For this review, take the finished solid that the model builds, in its own axes (mm). Face numbers are marked on the shaded views. A direction names the side the tool comes from. Give positions to 0.01 mm unless a question says otherwise; leave off trailing zeros. Loops run counter-clockwise (first coordinate to the right, second up) from the corner with the lowest first, then second, coordinate; pieces in that order, holes last. Notation, with made-up numbers: (4.5, 69.5) - (30.5, 69.5) arc R25 cw to (30.5, 81.5) - close; hole circle Ø2 at (23, 86). An arc over 180 degrees is marked (long way). Put each result on its own line as item: value. Start each with the question number.
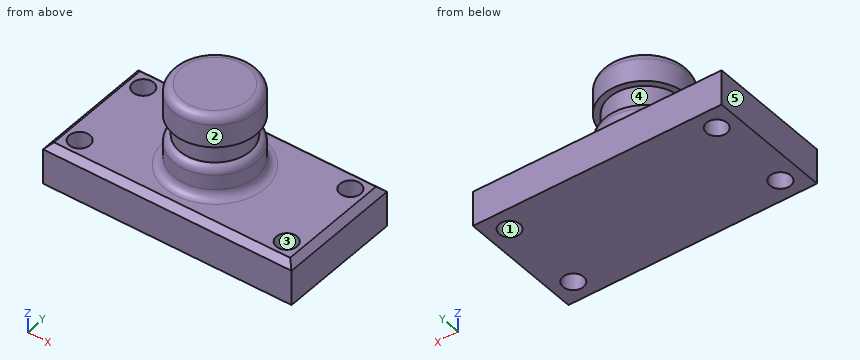
from build123d import *

# Parameters (mm, degrees)
F0_W     = 152.4
F0_H     = 76.2
F1_DEPTH = 25.4
F2_R     = 6.35
F3_DEPTH = 25.401
F4_SIZE  = 3.81


# Not quite as in the source:
# - a fillet or chamfer that OpenCascade refuses, or shapes differently, is made with other operations: its cross-section is extruded or revolved along the edge and cut away or added


with BuildPart() as f1:
    # F0 (on Top) → F1 (new body)
    with BuildSketch(Plane.XY):
        Rectangle(F0_W, F0_H)
    extrude(amount=F1_DEPTH)

    # F2 (on face) → F3 (cut, through all)
    with BuildSketch(Plane.XY.offset(25.4)):
        with Locations((-63.5, 25.4)):
            Circle(F2_R)
        with Locations((63.5, 25.4)):
            Circle(F2_R)
        with Locations((63.5, -25.4)):
            Circle(F2_R)
        with Locations((-63.5, -25.4)):
            Circle(F2_R)
    extrude(amount=-F3_DEPTH, mode=Mode.SUBTRACT)

    # F4
    f4_edges = [f1.edges().sort_by_distance(p)[0] for p in [
        (0, -38.1, 25.4),
        (-76.2, 0, 25.4),
        (0, 38.1, 25.4),
        (76.2, 0, 25.4),
    ]]
    chamfer(f4_edges, length=F4_SIZE)

    # F5 (on Front) → F6 (revolve)
    with BuildSketch(Plane.XZ):
        Polygon((0, 76.2), (0, 25.4), (25.4, 25.4), (25.4, 44.45), (21.59, 44.45), (21.59, 57.15), (25.4, 57.15), (25.4, 76.2), align=None)
    revolve(axis=Axis((0, 0, 50.8), (0, 0, 1)))

    # F7: fillet of radius 5.08 on 3 edges, made by hand

    # F7_s1 → F7_t2 (revolve)
    with BuildSketch(Plane.XZ):
        with BuildLine():
            ThreePointArc((30.48, 25.4), (26.8878975516, 26.8878975516), (25.4, 30.48))
            Line((25.4, 30.48), (25.4, 25.4))
            Line((25.4, 25.4), (30.48, 25.4))
        make_face()
    revolve(axis=Axis((0, 0, 25.4), (0, 0, 1)))

    # F7_s3 → F7_t4 (revolve, cut)
    with BuildSketch(Plane.XZ):
        with BuildLine():
            ThreePointArc((25.4, 39.5313111503), (24.3360926284, 42.6421631237), (21.59, 44.45))
            Line((21.59, 44.45), (25.4, 44.45))
            Line((25.4, 44.45), (25.4, 39.5313111503))
        make_face()
    revolve(axis=Axis((0, 0, 44.45), (0, 0, 1)), mode=Mode.SUBTRACT)

    # F7_s5 → F7_t6 (revolve, cut)
    with BuildSketch(Plane.XZ):
        with BuildLine():
            ThreePointArc((25.4, 71.12), (23.9121024484, 74.7121024484), (20.32, 76.2))
            Line((20.32, 76.2), (25.4, 76.2))
            Line((25.4, 76.2), (25.4, 71.12))
        make_face()
    revolve(axis=Axis((0, 0, 76.2), (0, 0, 1)), mode=Mode.SUBTRACT)


solid = f1.part
1) Machinability: for the marked faces 1 and 2, which of the approach directions +Z, -Z, +X, -X, +Y, -Y give a long, thin tool a straight path to every point of the face, cutting with its end or side? Answer none if there is none.
2) Take a section at D-D on z = 36.5. State the section outline as (x, y) points.
3) Take a section at B-B on y = 0. State the section outline as (x, z) points, and give its area (3 significant figures).
4) Insertion check: P1, Ø20.5, axis at x = 30, y = -9.5, coming from the +Z side; P2, Ø11.5, axis at x = 63.5, y = -25.4, coming from the -Z side (3 decimals); P3, Ø8, axis at x = -0.5, z = 62, coming from the -Y side; P4, Ø20.5, axis at x = -63.5, y = -25.4, coming from the +Z side. Each pin has a flat end and moves straight along its axis. Give the tip position at first contact, or say it passes through.
5) Take a section at C-C on x = 0. State the section outline as (y, z) points.
6) Take a section at A-A on x = 63.5. State the section outline as (y, z) points, and give its area (3 significant figures).
7) Wall thickness on probe 1 along Y at (x, z) = (-63.5, 11); probe 2 along X at (y, z) = (-25, 18); probe 3 along Y at (x, z) = (61.5, 15.5): over which ranges is each line inside the solid? List them lowest first.
8) Mouldability with a two-part tool opening along Y and no side actions: class the marked faces 3, 4 and 5 as released by +Y, released by -Y, zero draft, split by the parting line, or undercut.
Answers follow:
1. face 1: +Z, -Z
1. face 2: +Z
2. outline: circle Ø50.8 at (0, 0)
3. outline: (-76.2, 0) - (76.2, 0) - (76.2, 21.59) - (72.39, 25.4) - (30.48, 25.4) arc R5.08 cw to (25.4, 30.48) - (25.4, 39.53) arc R5.08 ccw to (21.59, 44.45) - (21.59, 57.15) - (25.4, 57.15) - (25.4, 71.12) arc R5.08 ccw to (20.32, 76.2) - (-20.32, 76.2) arc R5.08 ccw to (-25.4, 71.12) - (-25.4, 57.15) - (-21.59, 57.15) - (-21.59, 44.45) arc R5.08 ccw to (-25.4, 39.53) - (-25.4, 30.48) arc R5.08 cw to (-30.48, 25.4) - (-72.39, 25.4) - (-76.2, 21.59) - close
3. area: 6,330 mm2
4. P1: z = 76.12
4. P2: through
4. P3: y = -25.4
4. P4: z = 25.4
5. outline: (-38.1, 0) - (38.1, 0) - (38.1, 21.59) - (34.29, 25.4) - (30.48, 25.4) arc R5.08 cw to (25.4, 30.48) - (25.4, 39.53) arc R5.08 ccw to (21.59, 44.45) - (21.59, 57.15) - (25.4, 57.15) - (25.4, 71.12) arc R5.08 ccw to (20.32, 76.2) - (-20.32, 76.2) arc R5.08 ccw to (-25.4, 71.12) - (-25.4, 57.15) - (-21.59, 57.15) - (-21.59, 44.45) arc R5.08 ccw to (-25.4, 39.53) - (-25.4, 30.48) arc R5.08 cw to (-30.48, 25.4) - (-34.29, 25.4) - (-38.1, 21.59) - close
6. outline: (-38.1, 0) - (-31.75, 0) - (-31.75, 25.4) - (-34.29, 25.4) - (-38.1, 21.59) - close; (-19.05, 0) - (19.05, 0) - (19.05, 25.4) - (-19.05, 25.4) - close; (31.75, 0) - (38.1, 0) - (38.1, 21.59) - (34.29, 25.4) - (31.75, 25.4) - close
6. area: 1,280 mm2
7. probe 1: -38.1 to -31.75, -19.05 to 19.05, 31.75 to 38.1
7. probe 2: -76.2 to -69.84, -57.16 to 57.16, 69.84 to 76.2
7. probe 3: -38.1 to -31.43, -19.37 to 19.37, 31.43 to 38.1
8. face 3: undercut
8. face 4: split by the parting line
8. face 5: zero draft
